For this review, take the finished solid that the model builds, in its own axes (mm). Coordinates: 2 decimals unless noted, no trailing zeros. Order: outer loops, then holes, each group sorted by start corner. A loop starts at its lowest first (then second) coordinate and runs counter-clockwise, first axis right, second up. Notation, with made-up numbers: (81.25, 17.25) -> (102.25, 17.25) arc R29 cw to (102.25, 50.25) -> close; hole circle Ø9 at (39.25, 58.5). An arc over 180 degrees is marked (long way). Write item = value, one per line. Start each with the question number.
1) Wall thickness on probe 1 along X at (y, z) = (-63, 182); probe 2 along Z at (x, y) = (220, -208); probe 3 along Y at (x, z) = (71.5, 105.5): over which ranges is each line inside the solid? List them lowest first. Write a range as [from, to].
2) Consider section B-B on y = -38.5. Give the boundary of the cut face in (x, z).
3) Consider section A-A on z = 119.5. Give the boundary of the cut face in (x, y).
4) Insertion check: pin 1 Ø1 at (x, z) = (-96, 155) entering from +Y; pin 2 Ø6 at (y, z) = (-32.5, 203) entering from +X; pin 3 Ø6 at (y, z) = (100.5, 48.5) entering from +X. Each pin has a flat end and moves straight along its axis. Give the tip position at first contact, or say it passes through.
from build123d import *

# Parameters (mm, degrees)
F0_W     = 550
F0_H     = 550
F1_DEPTH = 246.83
F2_SIZE2 = 246.82999
F2_SIZE  = 274.99999
F4_DEPTH = 275


# Not quite as in the source:
# - a fillet or chamfer is up to 0.001 mm smaller than in the source, because OpenCascade refuses the exact size


with BuildPart() as f1:
    # F0 (on Top) → F1 (new body)
    with BuildSketch(Plane.XY):
        Rectangle(F0_W, F0_H)
    extrude(amount=F1_DEPTH)

    # F2 (size 275 and 246.83 in the source; OpenCascade refuses exactly that, so slightly less here)
    f2_edges = [f1.edges().sort_by_distance(p)[0] for p in [
        (0, -275, 246.83),
        (0, 275, 246.83),
    ]]
    f2_side = f1.faces().sort_by_distance((0, 0, 246.83))[0]
    chamfer(f2_edges, length=F2_SIZE, length2=F2_SIZE2, reference=f2_side)

    # F3 (on Front) → F4 (cut, symmetric)
    with BuildSketch(Plane.XZ):
        Polygon((-275, 246.83), (-275, 0), (0, 246.83), align=None)
        Polygon((275, 246.83), (0, 246.83), (275, 0), align=None)
    extrude(amount=F4_DEPTH, both=True, mode=Mode.SUBTRACT)


solid = f1.part
Answer sheet:
q1.probe_1 = [-72.23, 72.23]
q1.probe_2 = [0, 49.37]
q1.probe_3 = [-157.46, 157.46]
q2.outline = (-275, 0) -> (275, 0) -> (38.5, 212.27) -> (-38.5, 212.27) -> close
q3.outline = (-141.86, -141.86) -> (141.86, -141.86) -> (141.86, 141.86) -> (-141.86, 141.86) -> close
q4.pin_1 = 102.87
q4.pin_2 = 52.17
q4.pin_3 = 224.31
